Design review of the part built by this model. Coordinates are the model's own, in mm. A direction names the side the tool comes from. Round coordinates to 2 decimals unless told otherwise and drop trailing zeros. Loops run counter-clockwise (first coordinate to the right, second up) from the corner with the lowest first, then second, coordinate; pieces in that order, holes last. Notation, with made-up numbers: (87.25, 2.25) - (140.25, 2.25) arc R16 cw to (140.25, 22.25) - close; hole circle Ø5 at (79.5, -28.5). An arc over 180 degrees is marked (long way). One line per question, with ' | ' between items. Start each with the question number.
Autodesk Inventor part; units mm, degrees
ref_plane "YZ Plane" through (0, 0, 0) normal (1, 0, 0) x (0, 1, 0)
ref_plane "XZ Plane" through (0, 0, 0) normal (0, 1, 0) x (-1, 0, 0)
ref_plane "XY Plane" through (0, 0, 0) normal (0, 0, 1) x (1, 0, 0)
sketch "스케치1" plane through (0, 0, 0) normal (0, 0, 1) x (1, 0, 0)
  line L0 (0, 0) -> (22, 0)
  line L1 (0, 6) -> (22, 6)
  line L2 (0, -76) -> (22, -76)
  line L3 (0, -70) -> (22, -70)
  line L4 (0, 6) -> (50, 6)
  line L5 (50, 6) -> (50, -76)
  line L6 (50, -76) -> (0, -76)
  line L7 (0, -76) -> (0, 6)
  line L8 (22, 0) -> (28, 0)
  line L9 (28, 0) -> (28, 6)
  line L10 (22, 6) -> (22, 0)
  line L11 (22, -76) -> (28, -76)
  line L12 (28, -76) -> (28, -70)
  line L13 (22, -70) -> (22, -76)
  line L14 (22, 0) -> (22, 6)
  line L15 (28, 6) -> (22, 6)
  line L16 (28, -70) -> (22, -70)
  line L17 (22, -76) -> (22, -70)
  line L18 (0, -76) -> (0, -70)
  line L19 (0, 0) -> (0, 6)
  line L20 (22, 6.2) -> (28.2, 6.2)
  line L21 (28.2, 6.2) -> (28.2, -0.2)
  line L22 (28.2, -0.2) -> (22, -0.2)
  line L23 (21.8, 6) -> (21.8, 0)
  line L24 (21.8, 0) -> (21.8, -0.2)
  line L25 (21.8, -0.2) -> (22, -0.2)
  line L26 (21.8, 6) -> (21.8, 6.2)
  line L27 (21.8, 6.2) -> (22, 6.2)
  line L28 (50, -35) -> (45, -35)
  line L29 (22, -70) -> (28, -70)
  line L30 (28, -70) -> (28, -76)
  line L31 (22, -76) -> (22, -70)
  line L32 (22, -70) -> (22, -76)
  line L33 (28, -76) -> (22, -76)
  line L34 (22, -76.2) -> (28.2, -76.2)
  line L35 (28.2, -76.2) -> (28.2, -69.8)
  line L36 (28.2, -69.8) -> (22, -69.8)
  line L37 (21.8, -76) -> (21.8, -70)
  line L38 (21.8, -70) -> (21.8, -69.8)
  line L39 (21.8, -69.8) -> (22, -69.8)
  line L40 (21.8, -76) -> (21.8, -76.2)
  line L41 (21.8, -76.2) -> (22, -76.2)
  circle A0 centre (28.2, -0.2) radius 1
  circle A1 centre (21.8, -0.2) radius 1
  circle A2 centre (28.2, 6.2) radius 1
  circle A3 centre (21.8, 6.2) radius 1
  circle A4 centre (28.2, -69.8) radius 1
  circle A5 centre (21.8, -69.8) radius 1
  circle A6 centre (28.2, -76.2) radius 1
  circle A7 centre (21.8, -76.2) radius 1
  point P0 (50, -70)
  point P1 (50, 0)
  point P2 (28.2, -76)
  point P3 (28.2, 6)
  dimension "d7" = 0.2
  dimension "d8" = 0.2
  dimension "d9" = 2
  dimension "d10" = 2
  dimension "d11" = 2
  dimension "d12" = 2
extrude "돌출1" add sketch "스케치1" along normal blind 6 contours L24 L25 L22 A1 L0 | L0 A1 L23 | A1 L22 A0 L21 A2 L4 L5 L6 A6 L35 A4 L36 A5 L3 L7 L0 | L0 L7 L1 A3 L23 A1 | A3 L1 L23 | L3 A5 L37 A7 L2 L7 | L22 L21 A0 | A5 L36 L39 L38 L3 | L3 L37 A5 | A7 L37 L2 | L21 L4 A2 | A4 L35 L36 | L2 L6 A7 L34 L41 L40 | A7 L6 A6 L34 | A6 L6 L35 L34 | A6 L6 L35 picked at (27.8, -76.1333)
sketch "스케치2" plane through (0, 0, 6) normal (0, 0, 1) x (1, 0, 0)
  circle A0 centre (45.8, -4.2) radius 1.6
  circle A1 centre (45.8, -65.8) radius 1.6
  circle A2 centre (4.2, -4.2) radius 1.6
  circle A3 centre (4.2, -65.8) radius 1.6
  line L0 (50, -70) -> (50, 0)
  line L1 (50, 0) -> (0, 0)
  line L2 (0, 0) -> (0, -70)
  line L3 (0, -70) -> (50, -70)
  line L4 (28.4609, -19.5584) -> (28.4609, -20.3691)
  line L5 (28.4609, -20.3691) -> (23.0826, -20.3691)
  line L6 (23.0826, -20.3691) -> (23.0826, -22.4156)
  line L7 (23.0826, -22.4156) -> (22.3609, -22.4156)
  line L8 (22.3609, -22.4156) -> (22.3609, -17.5118)
  line L9 (22.3609, -17.5118) -> (23.0826, -17.5118)
  line L10 (23.0826, -17.5118) -> (23.0826, -19.5584)
  line L11 (23.0826, -19.5584) -> (28.4609, -19.5584)
  spline S0 degree 2 poles (28.0259, -26.6668) (28.3126, -26.9584) (28.5894, -27.7296) (28.5894, -28.2931) knots 0 0 0 1 2 2 2
  spline S1 degree 2 poles (28.5894, -28.2931) (28.5894, -28.8319) (28.3076, -29.6328) (28.0259, -29.9145) knots 0 0 0 1 2 2 2
  spline S2 degree 2 poles (28.0259, -29.9145) (27.7095, -30.2358) (26.8197, -30.4978) (26.1672, -30.4978) knots 0 0 0 1 2 2 2
  line L12 (26.1672, -30.4978) -> (22.3609, -30.4978)
  line L13 (22.3609, -30.4978) -> (22.3609, -29.6871)
  line L14 (22.3609, -29.6871) -> (26.1672, -29.6871)
  spline S3 degree 2 poles (26.1672, -29.6871) (26.5923, -29.6871) (27.1657, -29.5784) (27.3981, -29.4251) knots 0 0 0 1 2 2 2
  spline S4 degree 2 poles (27.3981, -29.4251) (27.6452, -29.262) (27.8973, -28.6985) (27.8973, -28.2931) knots 0 0 0 1 2 2 2
  spline S5 degree 2 poles (27.8973, -28.2931) (27.8973, -27.9125) (27.6452, -27.3193) (27.3981, -27.1562) knots 0 0 0 1 2 2 2
  spline S6 degree 2 poles (27.3981, -27.1562) (27.1657, -27.0029) (26.5972, -26.8942) (26.187, -26.8942) knots 0 0 0 1 2 2 2
  line L15 (26.187, -26.8942) -> (22.3609, -26.8942)
  line L16 (22.3609, -26.8942) -> (22.3609, -26.0835)
  line L17 (22.3609, -26.0835) -> (26.1672, -26.0835)
  spline S7 degree 2 poles (26.1672, -26.0835) (26.8049, -26.0835) (27.7144, -26.3405) (28.0259, -26.6668) knots 0 0 0 1 2 2 2
  line L18 (27.838, -41.6696) -> (28.4609, -41.6696)
  line L19 (28.4609, -41.6696) -> (28.4609, -44.0325)
  line L20 (28.4609, -44.0325) -> (27.838, -44.0325)
  line L21 (27.838, -44.0325) -> (27.838, -43.2564)
  line L22 (27.838, -43.2564) -> (22.9837, -43.2564)
  line L23 (22.9837, -43.2564) -> (22.9837, -44.0325)
  line L24 (22.9837, -44.0325) -> (22.3609, -44.0325)
  line L25 (22.3609, -44.0325) -> (22.3609, -41.6696)
  line L26 (22.3609, -41.6696) -> (22.9837, -41.6696)
  line L27 (22.9837, -41.6696) -> (22.9837, -42.4457)
  line L28 (22.9837, -42.4457) -> (27.838, -42.4457)
  line L29 (27.838, -42.4457) -> (27.838, -41.6696)
  spline S8 degree 2 poles (28.3917, -45.3623) (28.4806, -45.6292) (28.5696, -46.084) (28.5696, -46.4498) knots 0 0 0 1 2 2 2
  spline S9 degree 2 poles (28.5696, -46.4498) (28.5696, -47.043) (28.1692, -48.0464) (27.7688, -48.4123) knots 0 0 0 1 2 2 2
  spline S10 degree 2 poles (27.7688, -48.4123) (27.3733, -48.7781) (26.187, -49.1785) (25.4158, -49.1785) knots 0 0 0 1 2 2 2
  spline S11 degree 2 poles (25.4158, -49.1785) (24.6496, -49.1785) (23.5126, -48.7879) (23.0925, -48.4172) knots 0 0 0 1 2 2 2
  spline S12 degree 2 poles (23.0925, -48.4172) (22.6822, -48.0514) (22.2521, -47.0529) (22.2521, -46.4349) knots 0 0 0 1 2 2 2
  spline S13 degree 2 poles (22.2521, -46.4349) (22.2521, -46.1285) (22.3411, -45.5896) (22.4103, -45.3623) knots 0 0 0 1 2 2 2
  spline S14 degree 2 poles (22.4103, -45.3623) (22.4746, -45.1645) (22.6575, -44.7542) (22.7662, -44.5516) knots 0 0 0 1 2 2 2
  line L30 (22.7662, -44.5516) -> (23.745, -44.5516)
  line L31 (23.745, -44.5516) -> (23.745, -44.6158)
  spline S15 degree 2 poles (23.745, -44.6158) (23.6461, -44.7246) (23.3693, -45.0607) (23.2358, -45.3029) knots 0 0 0 1 2 2 2
  spline S16 degree 2 poles (23.2358, -45.3029) (23.1073, -45.5353) (22.9442, -46.084) (22.9442, -46.4399) knots 0 0 0 1 2 2 2
  spline S17 degree 2 poles (22.9442, -46.4399) (22.9442, -46.8304) (23.2655, -47.5274) (23.572, -47.7894) knots 0 0 0 1 2 2 2
  spline S18 degree 2 poles (23.572, -47.7894) (23.8834, -48.0464) (24.8276, -48.3332) (25.4158, -48.3332) knots 0 0 0 1 2 2 2
  spline S19 degree 2 poles (25.4158, -48.3332) (26.0436, -48.3332) (26.9482, -48.0316) (27.2596, -47.7696) knots 0 0 0 1 2 2 2
  spline S20 degree 2 poles (27.2596, -47.7696) (27.5612, -47.5126) (27.8677, -46.8255) (27.8677, -46.4399) knots 0 0 0 1 2 2 2
  spline S21 degree 2 poles (27.8677, -46.4399) (27.8677, -46.0889) (27.6947, -45.4908) (27.5661, -45.2584) knots 0 0 0 1 2 2 2
  spline S22 degree 2 poles (27.5661, -45.2584) (27.4376, -45.036) (27.1707, -44.7048) (27.0767, -44.6109) knots 0 0 0 1 2 2 2
  line L32 (27.0767, -44.6109) -> (27.0767, -44.5516)
  line L33 (27.0767, -44.5516) -> (28.0456, -44.5516)
  spline S23 degree 2 poles (28.0456, -44.5516) (28.1396, -44.7542) (28.3126, -45.1101) (28.3917, -45.3623) knots 0 0 0 1 2 2 2
  line L34 (25.8063, -38.1154) -> (28.4609, -35.9453)
  line L35 (28.4609, -35.9453) -> (28.4609, -36.9982)
  line L36 (28.4609, -36.9982) -> (26.0337, -38.9261)
  line L37 (26.0337, -38.9261) -> (26.0337, -39.8554)
  line L38 (26.0337, -39.8554) -> (28.4609, -39.8554)
  line L39 (28.4609, -39.8554) -> (28.4609, -40.6661)
  line L40 (28.4609, -40.6661) -> (22.3609, -40.6661)
  line L41 (22.3609, -40.6661) -> (22.3609, -39.0942)
  spline S24 degree 2 poles (22.3609, -39.0942) (22.3609, -38.5702) (22.4746, -37.8633) (22.6822, -37.542) knots 0 0 0 1 2 2 2
  spline S25 degree 2 poles (22.6822, -37.542) (22.8898, -37.2207) (23.5374, -36.8499) (24.0169, -36.8499) knots 0 0 0 1 2 2 2
  spline S26 degree 2 poles (24.0169, -36.8499) (24.6842, -36.8499) (25.5888, -37.5321) (25.8063, -38.1154) knots 0 0 0 1 2 2 2
  spline S27 degree 2 poles (28.3917, -31.9907) (28.4806, -32.2576) (28.5696, -32.7124) (28.5696, -33.0782) knots 0 0 0 1 2 2 2
  spline S28 degree 2 poles (28.5696, -33.0782) (28.5696, -33.6714) (28.1692, -34.6749) (27.7688, -35.0407) knots 0 0 0 1 2 2 2
  spline S29 degree 2 poles (27.7688, -35.0407) (27.3733, -35.4065) (26.187, -35.8069) (25.4158, -35.8069) knots 0 0 0 1 2 2 2
  spline S30 degree 2 poles (25.4158, -35.8069) (24.6496, -35.8069) (23.5126, -35.4164) (23.0925, -35.0456) knots 0 0 0 1 2 2 2
  spline S31 degree 2 poles (23.0925, -35.0456) (22.6822, -34.6798) (22.2521, -33.6813) (22.2521, -33.0634) knots 0 0 0 1 2 2 2
  spline S32 degree 2 poles (22.2521, -33.0634) (22.2521, -32.7569) (22.3411, -32.2181) (22.4103, -31.9907) knots 0 0 0 1 2 2 2
  spline S33 degree 2 poles (22.4103, -31.9907) (22.4746, -31.793) (22.6575, -31.3827) (22.7662, -31.18) knots 0 0 0 1 2 2 2
  line L42 (22.7662, -31.18) -> (23.745, -31.18)
  line L43 (23.745, -31.18) -> (23.745, -31.2443)
  spline S34 degree 2 poles (23.745, -31.2443) (23.6461, -31.353) (23.3693, -31.6892) (23.2358, -31.9314) knots 0 0 0 1 2 2 2
  spline S35 degree 2 poles (23.2358, -31.9314) (23.1073, -32.1637) (22.9442, -32.7124) (22.9442, -33.0683) knots 0 0 0 1 2 2 2
  spline S36 degree 2 poles (22.9442, -33.0683) (22.9442, -33.4588) (23.2655, -34.1558) (23.572, -34.4178) knots 0 0 0 1 2 2 2
  spline S37 degree 2 poles (23.572, -34.4178) (23.8834, -34.6749) (24.8276, -34.9616) (25.4158, -34.9616) knots 0 0 0 1 2 2 2
  spline S38 degree 2 poles (25.4158, -34.9616) (26.0436, -34.9616) (26.9482, -34.6601) (27.2596, -34.3981) knots 0 0 0 1 2 2 2
  spline S39 degree 2 poles (27.2596, -34.3981) (27.5612, -34.141) (27.8677, -33.4539) (27.8677, -33.0683) knots 0 0 0 1 2 2 2
  spline S40 degree 2 poles (27.8677, -33.0683) (27.8677, -32.7174) (27.6947, -32.1192) (27.5661, -31.8869) knots 0 0 0 1 2 2 2
  spline S41 degree 2 poles (27.5661, -31.8869) (27.4376, -31.6644) (27.1707, -31.3332) (27.0767, -31.2393) knots 0 0 0 1 2 2 2
  line L44 (27.0767, -31.2393) -> (27.0767, -31.18)
  line L45 (27.0767, -31.18) -> (28.0456, -31.18)
  spline S42 degree 2 poles (28.0456, -31.18) (28.1396, -31.3827) (28.3126, -31.7386) (28.3917, -31.9907) knots 0 0 0 1 2 2 2
  line L46 (27.838, -22.7962) -> (28.4609, -22.7962)
  line L47 (28.4609, -22.7962) -> (28.4609, -25.1591)
  line L48 (28.4609, -25.1591) -> (27.838, -25.1591)
  line L49 (27.838, -25.1591) -> (27.838, -24.383)
  line L50 (27.838, -24.383) -> (22.9837, -24.383)
  line L51 (22.9837, -24.383) -> (22.9837, -25.1591)
  line L52 (22.9837, -25.1591) -> (22.3609, -25.1591)
  line L53 (22.3609, -25.1591) -> (22.3609, -22.7962)
  line L54 (22.3609, -22.7962) -> (22.9837, -22.7962)
  line L55 (22.9837, -22.7962) -> (22.9837, -23.5723)
  line L56 (22.9837, -23.5723) -> (27.838, -23.5723)
  line L57 (27.838, -23.5723) -> (27.838, -22.7962)
extrude "돌출2" cut sketch "스케치2" against normal blind 6 contours A0 | A1 | A2 | A3
sketch "스케치3" plane through (0, 0, 6) normal (0, 0, 1) x (1, 0, 0)
  circle A0 centre (4.2, -65.8) radius 1.6
  circle A1 centre (45.8, -65.8) radius 1.6
  circle A2 centre (4.2, -4.2) radius 1.6
  circle A3 centre (45.8, -4.2) radius 1.6
  line L0 (50, 6) -> (28.2, 6)
  line L1 (21.8, 6) -> (0, 6)
  line L2 (0, 6) -> (0, -76)
  line L3 (0, -76) -> (21.8, -76)
  line L4 (50, -76) -> (50, 6)
  line L5 (28, 3) -> (45.8, 3)
  circle A4 centre (45.8, 3) radius 1.35
  line L6 (25, 0) -> (25, 3)
  circle A5 centre (4.2, 3) radius 1.35
  line L7 (50, -35) -> (44.45, -35)
  circle A6 centre (45.8, -73) radius 1.35
  circle A7 centre (4.2, -73) radius 1.35
  line L8 (28.2, -76.2) -> (28.2, -76)
  line L9 (28.2, -76) -> (21.8, -76)
  line L10 (21.8, -76) -> (21.8, -76.2)
  line L11 (21.8, -76.2) -> (28.2, -76.2)
  line L12 (28.2, -0.2) -> (21.8, -0.2)
  line L13 (21.8, -0.2) -> (21.8, 6)
  line L14 (21.8, -76) -> (21.8, -69.8)
  line L15 (21.8, -69.8) -> (28.2, -69.8)
  line L16 (28.2, -69.8) -> (28.2, -76)
  line L17 (28.2, -76) -> (50, -76)
  line L18 (28.2, 6) -> (28.2, -0.2)
  point P0 (0, 0)
  dimension "d4" = 2.7
extrude "돌출3" cut sketch "스케치3" against normal up to next contours A4 | L8 L11 L10 L9 | A5 | A6 | A7
properties part number "head_up"
1. The part is to be moulded in two halves that separate along X. For faces 1 (the face through (0, -36, 3)), 2 (the face through (50, -34, 3)), 3 (the face through (25, -0.2, 3)), say which applies: pulls with the +X half, pulls with the -X half, needs draft (parallel to the pull), parting line crosses it, or undercut.
2. Clearance check with flat-ended pins moving along their axes: P1, Ø3, axis at x = 45.8, y = -4.2, coming from the +Z side; P2, Ø3, axis at x = 25.5, z = 1.5, coming from the -Y side. State where each tip first meets the part, or that it passes through.
3. Take a section at C-C, the plane z = 2.9. Count the separate pieces of the cut face and the enclosed holes in it, then the cut area to 3 significant figures.
4. Take a section at B-B, the plane x = 45.8. Give the boundary of the cut face in (y, z).
5. Take a section at D-D, the plane y = 3. Give the boundary of the cut face in (x, z).
6. To check wall thickness, follow line 1 along Y through (x, z) = (4.2, 3.25); line 2 along X through (y, z) = (-65.8, 3.4); line 3 along X through (y, z) = (-73, 2.8). State the ranges of each line that lie inside material, in increasing order.
7. Take a section at A-A, the plane y = -65.8. Give the boundary of the cut face in (x, z).
8. Machinability: for faces 4 (the face through (4.82, -74.2, 3.04)), 5 (the face through (28.2, 3, 3)), 6 (the face through (25, -69.8, 3)), which of the approach directions +Z, -Z, +X, -X, +Y, -Y give a long, thin tool a straight path to every point of the face, cutting with its end or side? Answer none if there is none.
Answer list:
1) face 1: pulls with the -X half | face 2: pulls with the +X half | face 3: undercut
2) P1: passes through | P2: stops at y = -69.8
3) separate pieces: 1 | enclosed holes: 8 | area: 3,970 mm²
4) outline: (-76, 0) - (-74.35, 0) - (-74.35, 6) - (-76, 6) - close; (-71.65, 0) - (-67.4, 0) - (-67.4, 6) - (-71.65, 6) - close; (-64.2, 0) - (-5.8, 0) - (-5.8, 6) - (-64.2, 6) - close; (-2.6, 0) - (1.65, 0) - (1.65, 6) - (-2.6, 6) - close; (4.35, 0) - (6, 0) - (6, 6) - (4.35, 6) - close
5) outline: (0, 0) - (2.85, 0) - (2.85, 6) - (0, 6) - close; (5.55, 0) - (21.8, 0) - (21.8, 6) - (5.55, 6) - close; (28.2, 0) - (44.45, 0) - (44.45, 6) - (28.2, 6) - close; (47.15, 0) - (50, 0) - (50, 6) - (47.15, 6) - close
6) line 1: y = -76 to -74.35, -71.65 to -67.4, -64.2 to -5.8, -2.6 to 1.65, 4.35 to 6 | line 2: x = 0 to 2.6, 5.8 to 44.2, 47.4 to 50 | line 3: x = 0 to 2.85, 5.55 to 21.8, 28.2 to 44.45, 47.15 to 50
7) outline: (0, 0) - (2.6, 0) - (2.6, 6) - (0, 6) - close; (5.8, 0) - (44.2, 0) - (44.2, 6) - (5.8, 6) - close; (47.4, 0) - (50, 0) - (50, 6) - (47.4, 6) - close
8) face 4: +Z, -Z | face 5: +Z, -Z, +Y | face 6: +Z, -Z, -Y
